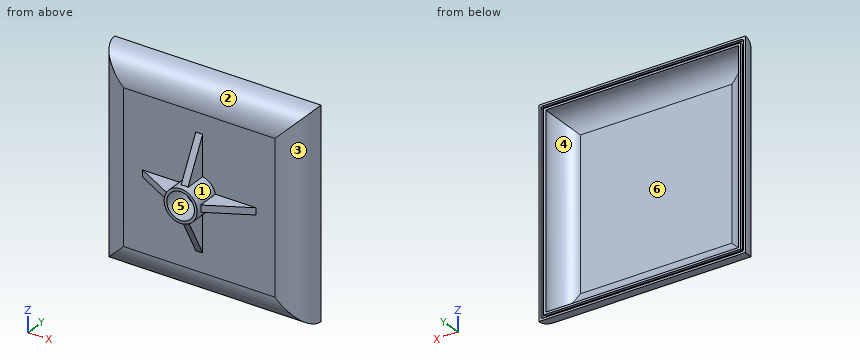
```python
from build123d import *

# Parameters (mm, degrees)
SKETCH1_W           = 150
SKETCH1_H           = 150
BOSS_EXTRUDE1_DEPTH = 20
FILLET8_R           = 20
SHELL1_T            = -5
SKETCH13_W          = 143
SKETCH13_H          = 143
CUT_EXTRUDE5_DEPTH  = 2
SKETCH14_R          = 12
SKETCH14_R_2        = 10
BOSS_EXTRUDE5_DEPTH = 20
RIB18_START         = -2.5
RIB18_DEPTH         = 5
CIRPATTERN1_COUNT   = 4


# Read off the part's stored shape, not the designer's step: Rib18
with BuildPart() as part:
    # Sketch1 → Boss-Extrude1 (new body)
    with BuildSketch(Plane(origin=(0, 0, 0), x_dir=(1, 0, 0), z_dir=(0, 1, 0))):
        with Locations((75, 75)):
            Rectangle(SKETCH1_W, SKETCH1_H)
    extrude(amount=BOSS_EXTRUDE1_DEPTH)

    # Fillet8
    fillet8_edges = [part.edges().sort_by_distance(p)[0] for p in [
        (75, 0, -150),
        (150, 0, -75),
        (75, 0, 0),
        (0, 0, -75),
    ]]
    fillet(fillet8_edges, radius=FILLET8_R - 0.0001)  # a hair under: the kernel refuses the full size

    # Shell1
    shell1_openings = [part.faces().sort_by_distance(p)[0] for p in [
        (75, 20, -75),
    ]]
    offset(amount=SHELL1_T, openings=shell1_openings)

    # Sketch13 → Cut-Extrude5 (cut)
    with BuildSketch(Plane(origin=(0, 20, 0), x_dir=(1, 0, 0), z_dir=(0, 1, 0))):
        with BuildLine():
            Line((1.5, 147.5), (1.5, 2.5))
            ThreePointArc((1.5, 2.5), (1.792893219, 1.792893219), (2.5, 1.5))
            Line((2.5, 1.5), (147.5, 1.5))
            ThreePointArc((147.5, 1.5), (148.207106781, 1.792893219), (148.5, 2.5))
            Line((148.5, 2.5), (148.5, 147.5))
            ThreePointArc((148.5, 147.5), (148.207106781, 148.207106781), (147.5, 148.5))
            Line((147.5, 148.5), (2.5, 148.5))
            ThreePointArc((2.5, 148.5), (1.792893219, 148.207106781), (1.5, 147.5))
        make_face()
        with Locations((75, 75)):
            Rectangle(SKETCH13_W, SKETCH13_H, mode=Mode.SUBTRACT)
    extrude(amount=-CUT_EXTRUDE5_DEPTH, mode=Mode.SUBTRACT)

    # Sketch14 → Boss-Extrude5 (add)
    with BuildSketch(Plane.XZ):
        with Locations(Location((75, -75, 0), (0, 0, 270))):
            Circle(SKETCH14_R)
        with Locations(Location((75, -75, 0), (0, 0, 270))):
            Circle(SKETCH14_R_2, mode=Mode.SUBTRACT)
    extrude(amount=BOSS_EXTRUDE5_DEPTH)

    # Rib18 outline → Rib18 (add)
    with BuildSketch(Plane.ZY.offset(-75).offset(RIB18_START)):
        Polygon((-85, 0), (-116.088549687, 0), (-86.736694594, -15.785154629), (-85, -16.719132826), align=None)
    rib18 = extrude(amount=RIB18_DEPTH)

    # CirPattern1: Rib18 ×4 about axis
    cirpattern1_axis = Axis((75, 0, -75), (0, 1, 0))
    for i in range(1, CIRPATTERN1_COUNT):
        add(rib18.rotate(cirpattern1_axis, i * 360 / CIRPATTERN1_COUNT))


solid = part.part
```
Read the model definition and answer for the solid it produces. Units are mm, in the model's axes. Face numbers are marked on the shaded views. A direction names the side the tool comes from. Coordinates: 2 decimals unless noted, no trailing zeros. Loops run counter-clockwise (first coordinate to the right, second up) from the corner with the lowest first, then second, coordinate; pieces in that order, holes last.
(1) Flat-ended cylindrical pins translate along their axes: pin 1 Ø1.6 at (y, z) = (18.5, -71) entering from +X; pin 2 Ø2 at (x, y) = (120, 4) entering from -Z; pin 3 Ø1.5 at (y, z) = (6, -50) entering from -X. Find the tip coordinate at first contact, or state that the pin passes through.
Solution:
pin 1: stops at x = 149.99
pin 2: stops at z = -143.23
pin 3: stops at x = 5.02
(2) The part is cut by section B-B (y = 9.5). Determine the outline of the cut face in (x, z), and give its area (3 significant figures).
Solution:
outline: (2.98, -147.02) - (147.02, -147.02) - (147.02, -2.98) - (2.98, -2.98) - close; hole (9.29, -140.71) - (140.71, -140.71) - (140.71, -9.29) - (9.29, -9.29) - close
area: 3,480 mm2
(3) Consider line 1 along Y through (x, z) = (101.5, -126); line 2 along Z through (x, y) = (49, -3.5); line 3 along X through (y, z) = (-4, -58). Determine where each line is inside the solid, lowest interval first.
Solution:
line 1: y = 0 to 5
line 2: z = -77.5 to -72.5
line 3: x = 72.5 to 77.5
(4) A tool of negligible diameter and unlimited length cuts with its end or side. For the marked faces 5 and 6, from which of +Z, -Z, +X, -X, +Y, -Y can it reach the whole face along a straight path? Write none if from no direction.
Solution:
face 5: -Y
face 6: +Y
(5) The mould has two halves that part along Z. Classify the marked faces 1, 2, 3 and 4: released by +Z, released by -Z, zero draft, split by the parting line, or undercut.
Solution:
face 1: split by the parting line
face 2: released by +Z
face 3: zero draft
face 4: undercut
